Here's how the part is built. I have some questions about the finished solid (model axes, mm). Face numbers are marked on the shaded views. A direction names the side the tool comes from. Give positions to 0.01 mm unless a question says otherwise; leave off trailing zeros. Loops run counter-clockwise (first coordinate to the right, second up) from the corner with the lowest first, then second, coordinate; pieces in that order, holes last.
Q1. For the marked faces 1, 2 and 3, which set-ups out of +Z, -Z, +X, -X, +Y, -Y let a thin tool reach every point of the face, with its end or its side?
Q2. If we section it at B-B (x = -5.5): Please give me the cut outline in (y, z).
Q3. If we section it at D-D (y = -19): Please give me the cut outline in (x, z).
Q4. If we section it at C-C (y = -3): Please give me the cut outline in (x, z), plus the area to 3 significant figures.
Q5. I need wall thicknesses on line 1 (Y direction, x = -13, z = 2.75); line 2 (X direction, y = 26.5, z = 6); line 3 (Y direction, x = -20.5, z = 0.5). Which ranges of each line are inside material? Lowest first, please.
Q6. We'd pull the mould along Y, two halves only. Please class the marked faces 4, 5 and 6: +Y half, -Y half, draft (parallel to the pull), parting line (faces both ways), or undercut.
Q7. Will these pins go through, and if not, where does the flat tip stop? P1, Ø0.8, axis at y = -18, z = -0.5, coming from the +X side; P2, Ø3, axis at y = -22.5, z = 5, coming from the -X side; P3, Ø1.3, axis at y = 35, z = 6.5, coming from the +X side.
Q8. If we section it at A-A (z = 3.75): Please give me the cut outline in (x, y).
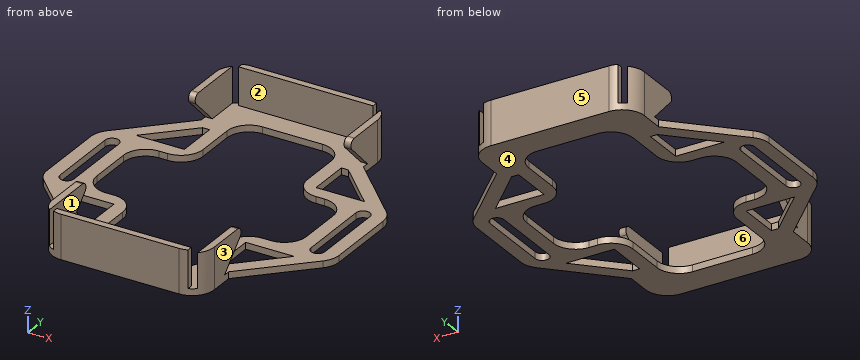
from build123d import *

# Parameters (mm, degrees)
F1_DEPTH        = 35.8775
F3_DEPTH        = 25.4
F4_W            = 1.5875
F4_H            = 8.9535
F5_DEPTH        = 9.525
F6_W            = 30.924
F6_H            = 1.5875
F5_FACE_W       = 1.5875
F5_FACE_H       = 8.9535
F7_DEPTH        = 8.636
F8_W            = 4.9497522414
F8_H            = 7.6485192403
F9_DEPTH        = 71.756
F10_W           = 23.939
F10_H           = 58.42
F11_DEPTH       = 1.525
F13_DEPTH       = 25.4
F14_W           = 12.1285
F14_H           = 20.175
F15_DEPTH       = 25.4
F16_F1_R        = 5.08
F16_F2_R        = 5.08
F16_S1_T1_DEPTH = 26.1520932665
F18_DEPTH       = 25.4
F20_DEPTH       = 1.5875
F22_DEPTH       = 1.5875
F23_R           = 1.27
F24_W           = 14.2291039228
F24_H           = 17.7929829806
F25_DEPTH       = 2.54


# Not quite as in the source:
# - a fillet or chamfer that OpenCascade refuses, or shapes differently, is made with other operations: its cross-section is extruded or revolved along the edge and cut away or added


with BuildPart() as f1:
    # F0 (on Front) → F1 (new body, symmetric)
    with BuildSketch(Plane.XZ):
        Polygon((17.875, 0.762), (-17.875, 0.762), (-18.637, 0.762), (-18.637, 0), (-18.637, -0.762), (18.637, -0.762), (18.637, 0), (18.637, 0.762), align=None)
    extrude(amount=F1_DEPTH, both=True)

    # F2 (on Front) → F3 (join, symmetric)
    with BuildSketch(Plane.XZ):
        Polygon((33.623, 0.762), (20.923, 0.762), (18.637, 0.762), (18.637, -0.762), (33.623, -0.762), align=None)
        Polygon((-18.637, 0.762), (-20.923, 0.762), (-33.623, 0.762), (-33.623, -0.762), (-18.637, -0.762), (-18.637, 0), align=None)
    extrude(amount=F3_DEPTH, both=True)

    # F4 (on face) → F5 (join)
    with BuildSketch(Plane(origin=(0, 0, -0.762), x_dir=(1, 0, 0), z_dir=(0, 0, -1))):
        with Locations((-17.84325, 31.40075)):
            Rectangle(F4_W, F4_H)
        with Locations((17.84325, 31.40075)):
            Rectangle(F4_W, F4_H)
        with Locations((-17.84325, -31.40075)):
            Rectangle(F4_W, F4_H)
        with Locations((17.84325, -31.40075)):
            Rectangle(F4_W, F4_H)
    extrude(amount=-F5_DEPTH)

    # F6 (on face) + F5_face (on face) → F7 (join)
    with BuildSketch(Plane.XY.offset(0.762)):
        with Locations((0, 35.08375)):
            Rectangle(F6_W, F6_H)
        with Locations((0, -35.08375)):
            Rectangle(F6_W, F6_H)
    with BuildSketch(Plane(origin=(-17.84325, 31.40075, 8.763), x_dir=(1, 0, 0), z_dir=(0, 0, 1))):
        Rectangle(F5_FACE_W, F5_FACE_H)
    extrude(amount=F7_DEPTH)

    # F8 (on face) → F9 (cut, through all)
    with BuildSketch(Plane(origin=(0, 35.8775, 0), x_dir=(-1, 0, 0), z_dir=(0, 1, 0))):
        with Locations((18.5586120933, 12.8226471134)):
            Rectangle(F8_W, F8_H)
    extrude(amount=-F9_DEPTH, mode=Mode.SUBTRACT)

    # F10 (on face) → F11 (cut, through all)
    with BuildSketch(Plane.XY.offset(0.762)):
        with BuildLine():
            ThreePointArc((-30.448, -8.5), (-28.8605, -10.0875), (-27.273, -8.5))
            Line((-27.273, -8.5), (-27.273, 8.5))
            ThreePointArc((-27.273, 8.5), (-28.8605, 10.0875), (-30.448, 8.5))
            Line((-30.448, 8.5), (-30.448, -8.5))
        make_face()
        with BuildLine():
            Line((27.273, 8.5), (27.273, -8.5))
            ThreePointArc((27.273, -8.5), (28.8605, -10.0875), (30.448, -8.5))
            Line((30.448, -8.5), (30.448, 8.5))
            ThreePointArc((30.448, 8.5), (28.8605, 10.0875), (27.273, 8.5))
        make_face()
        Rectangle(F10_W, F10_H)
    extrude(amount=-F11_DEPTH, mode=Mode.SUBTRACT)

    # F12 (on face) → F13 (cut)
    with BuildSketch(Plane.XY.offset(0.762)):
        Polygon((33.623, 25.4), (18.637, 25.4), (33.623, 10.414), align=None)
        Polygon((33.623, -10.414), (18.637, -25.4), (33.623, -25.4), align=None)
        Polygon((-18.637, 25.4), (-33.623, 25.4), (-33.623, 10.414), align=None)
        Polygon((-33.623, -10.414), (-33.623, -25.4), (-18.637, -25.4), align=None)
    extrude(amount=-F13_DEPTH, mode=Mode.SUBTRACT)

    # F14 (on face) → F15 (cut)
    with BuildSketch(Plane.XY.offset(0.762)):
        with Locations((-18.03375, 0)):
            Rectangle(F14_W, F14_H)
        with Locations((18.03375, 0)):
            Rectangle(F14_W, F14_H)
        Polygon((-15.1445, 16.4375), (-23.1093719395, 16.4375), (-26.2843719395, 13.2625), (-15.1445, 13.2625), align=None)
        Polygon((-19.9343719395, 19.6125), (-16.7593719395, 19.6125), (-15.1445, 19.6125), (-15.1445, 22.7875), (-16.7593719395, 22.7875), align=None)
        Polygon((16.7593719395, 19.6125), (19.9343719395, 19.6125), (16.7593719395, 22.7875), (15.1445, 22.7875), (15.1445, 19.6125), align=None)
        Polygon((23.1093719395, 16.4375), (15.1445, 16.4375), (15.1445, 13.2625), (26.2843719395, 13.2625), align=None)
        Polygon((26.2843719395, -13.2625), (15.1445, -13.2625), (15.1445, -16.4375), (23.1093719395, -16.4375), align=None)
        Polygon((16.7593719395, -22.7875), (19.9343719395, -19.6125), (16.7593719395, -19.6125), (15.1445, -19.6125), (15.1445, -22.7875), align=None)
        Polygon((-15.1445, -13.2625), (-26.2843719395, -13.2625), (-23.1093719395, -16.4375), (-15.1445, -16.4375), align=None)
        Polygon((-15.1445, -19.6125), (-16.7593719395, -19.6125), (-19.9343719395, -19.6125), (-16.7593719395, -22.7875), (-15.1445, -22.7875), align=None)
    extrude(amount=-F15_DEPTH, mode=Mode.SUBTRACT)

    # F16: fillet of radius 5.08 on 20 edges, made by hand

    # F16_f1
    f16_f1_edges = [f1.edges().sort_by_distance(p)[0] for p in [
        (-24.098, 10.0875, 0),
        (-24.098, -10.0875, 0),
        (-11.9695, 29.21, 0),
        (11.9695, 29.21, 0),
        (24.098, 10.0875, 0),
        (24.098, -10.0875, 0),
        (11.9695, -29.21, 0),
        (-11.9695, -29.21, 0),
    ]]
    fillet(f16_f1_edges, radius=F16_F1_R)

    # F16_f2
    f16_f2_edges = [f1.edges().sort_by_distance(p)[0] for p in [
        (-33.623, -10.414, 0),
        (-33.623, 10.414, 0),
        (-11.9695, -10.0875, 0),
        (-11.9695, 10.0875, 0),
        (11.9695, 10.0875, 0),
        (11.9695, -10.0875, 0),
        (33.623, -10.414, 0),
        (33.623, 10.414, 0),
        (18.637, 35.8775, 4.0005),
        (-18.637, 35.8775, 4.1181937466),
        (18.637, -35.8775, 4.0005),
        (-18.637, -35.8775, 4.0005),
    ]]
    fillet(f16_f2_edges, radius=F16_F2_R)

    # F16#s1: fillet of radius 5.08 on 1 edges, made by hand

    # F16_s1_s2 → F16_s1_t1 (cut)
    with BuildSketch(Plane.XY.offset(3.9469067335)):
        with BuildLine():
            ThreePointArc((-13.557, 35.8775), (-17.1491024484, 34.3896024484), (-18.637, 30.7975))
            Line((-18.637, 30.7975), (-18.637, 35.8775))
            Line((-18.637, 35.8775), (-13.557, 35.8775))
        make_face()
    extrude(amount=F16_S1_T1_DEPTH, mode=Mode.SUBTRACT)

    # F17 (on face) → F18 (cut)
    with BuildSketch(Plane.XY.offset(0.762)):
        Polygon((-15.1445, 19.6125), (-19.9343719395, 19.6125), (-23.1093719395, 16.4375), (-15.1445, 16.4375), align=None)
        Polygon((19.9343719395, 19.6125), (15.1445, 19.6125), (15.1445, 16.4375), (23.1093719395, 16.4375), align=None)
        Polygon((23.1093719395, -16.4375), (15.1445, -16.4375), (15.1445, -19.6125), (19.9343719395, -19.6125), align=None)
        Polygon((-15.1445, -16.4375), (-23.1093719395, -16.4375), (-19.9343719395, -19.6125), (-15.1445, -19.6125), align=None)
    extrude(amount=-F18_DEPTH, mode=Mode.SUBTRACT)

    # F19 (on face) → F20 (join)
    with BuildSketch(Plane.YZ.offset(18.637)):
        Polygon((18.923, 8.763), (26.924, 0.762), (26.924, 8.763), align=None)
        Polygon((-26.924, 8.763), (-26.924, 0.762), (-18.923, 8.763), align=None)
    extrude(amount=-F20_DEPTH)

    # F21 (on face) → F22 (join)
    with BuildSketch(Plane(origin=(-18.637, 0, 0), x_dir=(0, -1, 0), z_dir=(-1, 0, 0))):
        Polygon((18.923, 8.763), (26.924, 0.762), (26.924, 8.763), align=None)
        Polygon((-26.924, 8.9983874932), (-26.924, 0.762), (-18.6876125068, 8.9983874932), align=None)
    extrude(amount=-F22_DEPTH)

    # F23
    f23_edges = [f1.edges().sort_by_distance(p)[0] for p in [
        (-17.84325, 18.687613, 8.998387),
        (-17.84325, -18.923, 8.763),
        (17.84325, -18.923, 8.763),
        (17.84325, 18.923, 8.763),
    ]]
    fillet(f23_edges, radius=F23_R)

    # F24 (on face) → F25 (cut)
    with BuildSketch(Plane.XY.offset(17.399)):
        with Locations((-13.9599367976, 29.4290939346)):
            Rectangle(F24_W, F24_H)
    extrude(amount=-F25_DEPTH, mode=Mode.SUBTRACT)


solid = f1.part
Check sheet entries:
1. face 1: +Z, +Y, -Y
1. face 2: +Z
1. face 3: +Z, +X, -Y
2. outline: (-35.88, -0.76) - (-29.21, -0.76) - (-29.21, 0.76) - (-34.29, 0.76) - (-34.29, 9.4) - (-35.88, 9.4) - close; (29.21, -0.76) - (35.88, -0.76) - (35.88, 9.4) - (34.29, 9.4) - (34.29, 0.76) - (29.21, 0.76) - close
3. outline: (-25.04, -0.76) - (-20.55, -0.76) - (-20.55, 0.76) - (-25.04, 0.76) - close; (-15.14, -0.76) - (-11.97, -0.76) - (-11.97, 0.76) - (-15.14, 0.76) - close; (11.97, -0.76) - (15.14, -0.76) - (15.14, 0.76) - (11.97, 0.76) - close; (20.55, -0.76) - (25.04, -0.76) - (25.04, 0.76) - (20.55, 0.76) - close
4. outline: (-33.62, -0.76) - (-30.45, -0.76) - (-30.45, 0.76) - (-33.62, 0.76) - close; (-27.27, -0.76) - (-24.1, -0.76) - (-24.1, 0.76) - (-27.27, 0.76) - close; (24.1, -0.76) - (27.27, -0.76) - (27.27, 0.76) - (24.1, 0.76) - close; (30.45, -0.76) - (33.62, -0.76) - (33.62, 0.76) - (30.45, 0.76) - close
4. area: 19.4 mm2
5. line 1: y = -35.88 to -34.29, 34.29 to 35.88
5. line 2: x = -18.64 to -17.05, 17.05 to 18.64
5. line 3: y = -23.54 to -19.05, -13.26 to -9.87, 9.87 to 13.26, 19.05 to 23.54
6. face 4: draft
6. face 5: +Y half
6. face 6: undercut
7. P1: stops at x = 26.44
7. P2: stops at x = -18.64
7. P3: stops at x = 17.19
8. outline: (-18.64, -30.8) arc R5.08 ccw to (-17.05, -34.49) - (-17.05, -23.94) - (-18.64, -23.94) - close; (-18.64, 23.94) - (-17.05, 23.94) - (-17.05, 34.49) arc R5.08 ccw to (-18.64, 30.8) - close; (-15.46, -35.51) arc R5.08 ccw to (-13.56, -35.88) - (13.56, -35.88) arc R5.08 ccw to (15.46, -35.51) - (15.46, -34.29) - (-15.46, -34.29) - close; (-15.46, 34.29) - (15.46, 34.29) - (15.46, 35.51) arc R5.08 ccw to (13.56, 35.88) - (-13.56, 35.88) arc R5.08 ccw to (-15.46, 35.51) - close; (17.05, -34.49) arc R5.08 ccw to (18.64, -30.8) - (18.64, -23.94) - (17.05, -23.94) - close; (17.05, 23.94) - (18.64, 23.94) - (18.64, 30.8) arc R5.08 ccw to (17.05, 34.49) - close
